Part model, mm, in its own coordinate system. A direction names the side the tool comes from. Give positions to 0.01 mm unless a question says otherwise; leave off trailing zeros. Write each loop counter-clockwise with the first axis right and the second up, starting at its lowest first coordinate (ties: lowest second). Pieces come first, ordered by that corner, then holes. Notation, with made-up numbers: (-11.5, 7.5) - (13.5, 7.5) arc R15 cw to (13.5, 22.5) - close; hole circle Ø6 at (13.25, -19). An arc over 180 degrees is marked (long way). Answer as a JSON object with one key per item and string values. Group by question number.
```python
from build123d import *

# Parameters (mm, degrees)
SKETCH_1_R      = 1.65
EXTRUDE_1_DEPTH = 6
EXTRUDE_2_DEPTH = 75
EXTRUDE_START   = 25
SKETCH_3_R      = 2
EXTRUDE_3_DEPTH = 8
EXTRUDE_4_REACH = 93.669
SKETCH_5_W      = 45
SKETCH_5_H      = 8
EXTRUDE_START_2 = 33
SKETCH_6_W      = 8
SKETCH_6_H      = 8
EXTRUDE_5_DEPTH = 40
SKETCH_7_W      = 8
SKETCH_7_H      = 8
EXTRUDE_6_DEPTH = 50
SKETCH_8_W      = 8
SKETCH_8_H      = 17
EXTRUDE_7_DEPTH = 40


with BuildPart() as part:
    # Sketch 1 → Extrude 1 (new body)
    with BuildSketch(Plane(origin=(0, 0, 0), x_dir=(1, 0, 0), z_dir=(0, 1, 0))):
        Polygon((-10, 36), (-10, 10), (-36, 10), (-36, -10), (-10, -10), (-10, -36), (10, -36), (10, -10), (36, -10), (36, 10), (10, 10), (10, 36), align=None)
        with Locations(Location((0, 30, 0), (0, 0, 270))):
            Circle(SKETCH_1_R, mode=Mode.SUBTRACT)
        with Locations(Location((30, 0, 0), (0, 0, 270))):
            Circle(SKETCH_1_R, mode=Mode.SUBTRACT)
        with Locations(Location((0, -30, 0), (0, 0, 270))):
            Circle(SKETCH_1_R, mode=Mode.SUBTRACT)
        with Locations(Location((-30, 0, 0), (0, 0, 270))):
            Circle(SKETCH_1_R, mode=Mode.SUBTRACT)
    extrude(amount=EXTRUDE_1_DEPTH)

    # Sketch 2 → Extrude 2 (add)
    with BuildSketch(Plane(origin=(0, 0, 0), x_dir=(1, 0, 0), z_dir=(0, 1, 0))):
        with BuildLine():
            Line((-15, 20), (15, 20))
            ThreePointArc((15, 20), (18.535533906, 18.535533906), (20, 15))
            Line((20, 15), (20, -15))
            ThreePointArc((20, -15), (18.535533906, -18.535533906), (15, -20))
            Line((15, -20), (-15, -20))
            ThreePointArc((-15, -20), (-18.535533906, -18.535533906), (-20, -15))
            Line((-20, -15), (-20, 15))
            ThreePointArc((-20, 15), (-18.535533906, 18.535533906), (-15, 20))
        make_face()
    extrude(amount=EXTRUDE_2_DEPTH)


with BuildPart() as body_2:
    # Sketch 3 → Extrude 3 (new body)
    with BuildSketch(Plane(origin=(0, 75, 0), x_dir=(1, 0, 0), z_dir=(0, 1, 0)).offset(EXTRUDE_START)):
        Polygon((-38.5, -20), (18.5, -20), (18.5, 12), (10.5, 12), (10.5, -12), (-30.5, -12), (-30.5, 12), (-38.5, 12), align=None)
        with Locations(Location((-34.2, -4.9, 0), (0, 0, 90))):
            Circle(SKETCH_3_R, mode=Mode.SUBTRACT)
        with Locations(Location((-34.2, 4.9, 0), (0, 0, 90))):
            Circle(SKETCH_3_R, mode=Mode.SUBTRACT)
        with Locations(Location((14.2, -4.9, 0), (0, 0, 90))):
            Circle(SKETCH_3_R, mode=Mode.SUBTRACT)
        with Locations(Location((14.2, 4.9, 0), (0, 0, 90))):
            Circle(SKETCH_3_R, mode=Mode.SUBTRACT)
    extrude(amount=EXTRUDE_3_DEPTH)

    # Sketch 5 → Extrude 4 (add, up to next)
    with BuildSketch(Plane(origin=(0, 75, 0), x_dir=(1, 0, 0), z_dir=(0, 1, 0)), mode=Mode.PRIVATE) as extrude_4_sk1:
        with Locations((-7.5, -16)):
            Rectangle(SKETCH_5_W, SKETCH_5_H)
    extrude_4_tool1 = extrude(extrude_4_sk1.sketch, amount=EXTRUDE_4_REACH, mode=Mode.PRIVATE) - body_2.part

    add(part.part)  # Extrude 4 merges part
    add(extrude_4_tool1.solids().sort_by_distance((-7.5, 75, 16))[0])

    # Sketch 6 → Extrude 5 (add)
    with BuildSketch(Plane(origin=(0, 75, 0), x_dir=(1, 0, 0), z_dir=(0, 1, 0)).offset(EXTRUDE_START_2)):
        with Locations((22.5, 8)):
            Rectangle(SKETCH_6_W, SKETCH_6_H)
    extrude(amount=-EXTRUDE_5_DEPTH)

    # Sketch 7 → Extrude 6 (add)
    with BuildSketch(Plane(origin=(0, 108, 0), x_dir=(1, 0, 0), z_dir=(0, 1, 0))):
        with Locations((-34.5, 16)):
            Rectangle(SKETCH_7_W, SKETCH_7_H)
    extrude(amount=-EXTRUDE_6_DEPTH)

    # Sketch 8 → Extrude 7 (add)
    with BuildSketch(Plane.ZY.offset(38.5)):
        with Locations((-16, 66.5)):
            Rectangle(SKETCH_8_W, SKETCH_8_H)
    extrude(amount=-EXTRUDE_7_DEPTH)


solid = body_2.part
```
1) Mould opens along Z. For faces 6 (the flat face through (-38.5, 94, -13)), 7 (the cylindrical face through (31.636, 2.958, -0.215)), 8 (the flat face through (28, 3, 10)), 9 (the flat face through (0, 3, -36)) say: pulls with the +Z half, pulls with the -Z half, needs draft (parallel to the pull), parting line crosses it, or undercut.
2) Band-saw the part on D-D (x = -34.2). List the corners of the cut face in (y, z).
3) Band-saw the part on A-A (x = -26). List the corners of the cut face in (y, z), plus the area to 3 significant figures.
4) Probe line 1 (X direction, y = 3, z = 0); line 2 (Z direction, x = -34, y = 102); line 3 (X direction, y = 102.5, z = -4.9). List the from-to ranges inside material, lowest first.
5) Drop flat-ended pins along their axis: P1, Ø2, axis at y = 18.5, z = -22.5, coming from the -X side; P2, Ø6, axis at x = -9, y = 49.5, coming from the -Z side; P3, Ø10, axis at x = 2.5, y = 78, coming from the +Z side; P4, Ø2.5, axis at y = 79, z = -10, coming from the +X side. Give the stop position or say it passes through.
6) Band-saw the part on B-B (y = 83). List the corners of the cut face in (x, z), plus the area to 3 significant figures.
7) Band-saw the part on C-C (z = 0). List the corners of the cut face in (x, y), plus the area to 3 significant figures.
8) Which spindle directions (+Z, -Z, +X, -X, +Y, -Y) get a long thin tool onto all of the face, cutting with end or side? Do faces 1 (the cylindrical face through (-18, 37, 19)), 2 (the flat face through (10, 3, 28)), 3 (the flat face through (10.5, 104, 0)), 4 (the flat face through (18.5, 104, 8)), 5 (the flat face through (0, 6, -28)). Say none if no direction does.
Verdict:
{
 "1": {"face 6": "needs draft", "face 7": "undercut", "face 8": "pulls with the +Z half", "face 9": "pulls with the -Z half"},
 "2": {"outline": "(0, -10) - (6, -10) - (6, 10) - (0, 10) - close; (58, -20) - (108, -20) - (108, -6.9) - (100, -6.9) - (100, -12) - (58, -12) - close; (100, -2.9) - (108, -2.9) - (108, 2.9) - (100, 2.9) - close; (100, 6.9) - (108, 6.9) - (108, 20) - (100, 20) - close"},
 "3": {"outline": "(0, -10) - (6, -10) - (6, 10) - (0, 10) - close; (58, -20) - (75, -20) - (75, -12) - (58, -12) - close; (75, 12) - (108, 12) - (108, 20) - (75, 20) - close", "area": "520 mm2"},
 "4": {"line 1": "-36 to -31.65, -28.35 to 28.35, 31.65 to 36", "line 2": "-20 to -6.89, -2.91 to 2.91, 6.89 to 20", "line 3": "-38.5 to -36.2, -32.2 to -30.5, 10.5 to 12.2, 16.2 to 26.5"},
 "5": {"P1": "through", "P2": "z = -20", "P3": "z = 20", "P4": "x = 26.5"},
 "6": {"outline": "(-38.5, -20) - (-30.5, -20) - (-30.5, -12) - (-38.5, -12) - close; (-30, 12) - (15, 12) - (15, 20) - (-30, 20) - close; (18.5, -12) - (26.5, -12) - (26.5, -4) - (18.5, -4) - close", "area": "488 mm2"},
 "7": {"outline": "(-38.5, 100) - (-30.5, 100) - (-30.5, 108) - (-38.5, 108) - close; (-36, 0) - (-31.65, 0) - (-31.65, 6) - (-36, 6) - close; (-28.35, 0) - (28.35, 0) - (28.35, 6) - (20, 6) - (20, 75) - (-20, 75) - (-20, 6) - (-28.35, 6) - close; (10.5, 100) - (18.5, 100) - (18.5, 108) - (10.5, 108) - close; (31.65, 0) - (36, 0) - (36, 6) - (31.65, 6) - close", "area": "3,280 mm2"},
 "8": {"face 1": "+Z, -X, -Y", "face 2": "+Z, +X, +Y, -Y", "face 3": "-Z, +Y", "face 4": "+Z, +X, +Y", "face 5": "-Z, +X, -X, +Y"}
}
